Check sheet for the drawn part. Datum: minimum x, y, z corner. Units: mm. A direction names the side the tool comes from. Round coordinates to 2 decimals unless told otherwise and drop trailing zeros. Order: outer loops, then holes, each group sorted by start corner. A loop starts at its lowest first (then second) coordinate and runs counter-clockwise, first axis right, second up. Notation, with made-up numbers: (45.5, 22.5) -> (73.5, 22.5) arc R34 ccw to (73.5, 59.5) -> close; hole circle Ø2 at (53.25, -39.5). An arc over 180 degrees is marked (long way). Answer in a Markdown table with one row per item.
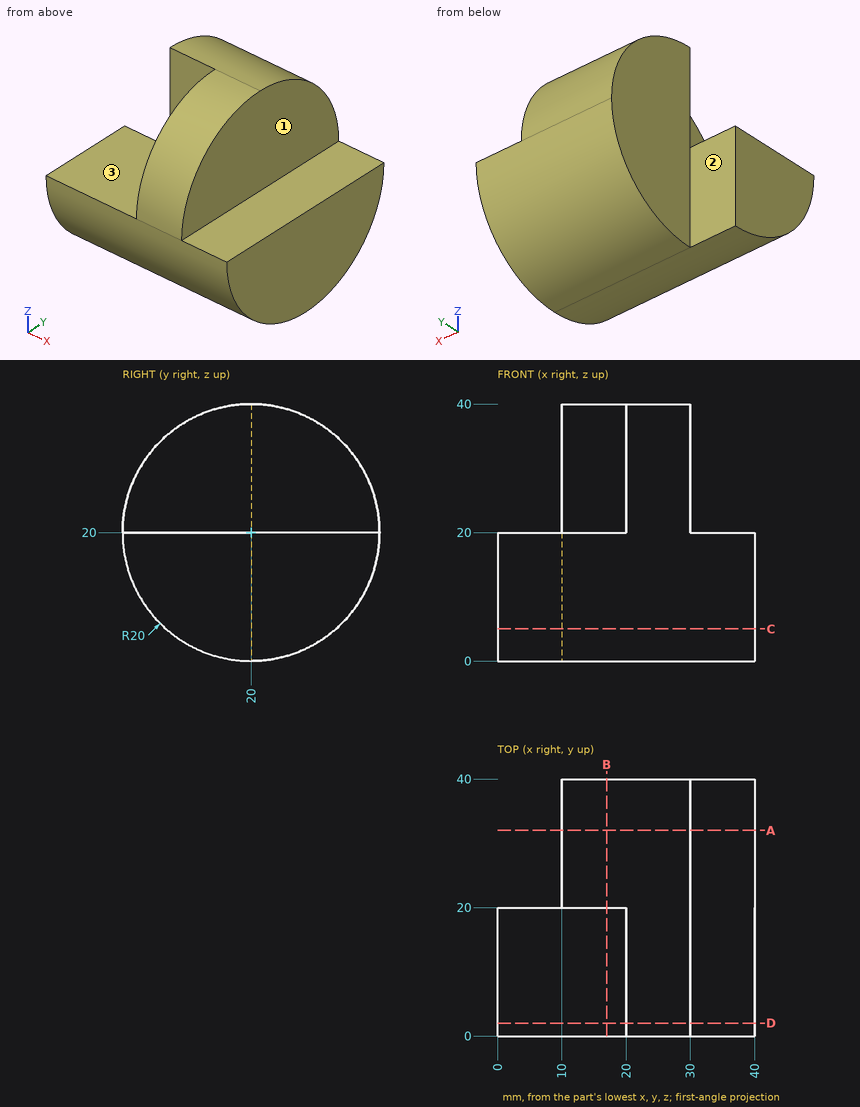
(1) Section check D-D on y = 2. Record the boundary of the cut face in (x, z).
Solutions:
| item | result |
|---|---|
| outline | (0, 11.28) -> (40, 11.28) -> (40, 20) -> (30, 20) -> (30, 28.72) -> (20, 28.72) -> (20, 20) -> (0, 20) -> close |
(2) Section check B-B on x = 17. Record the boundary of the cut face in (y, z), plus the area to 3 significant figures.
Solutions:
| item | result |
|---|---|
| outline | (0, 20) arc R20 ccw (long way) to (20, 40) -> (20, 20) -> close |
| area | 942 mm^2 |
(3) Section check C-C on z = 5. Record the boundary of the cut face in (x, y), plus the area to 3 significant figures.
Solutions:
| item | result |
|---|---|
| outline | (0, 6.77) -> (40, 6.77) -> (40, 33.23) -> (10, 33.23) -> (10, 20) -> (0, 20) -> close |
| area | 926 mm^2 |
(4) Scan lines: probe 1 along X at (y, z) = (35, 12); probe 2 along X at (y, z) = (6.5, 31); probe 3 along Y at (x, z) = (4, 15). Record each from-to range of solid material in increasing order. Write a range as from..to.
Solutions:
| item | result |
|---|---|
| probe 1 | 10..40 |
| probe 2 | 20..30 |
| probe 3 | 0.64..20 |
(5) Tool access check on the marked faces 1, 2 and 3. Record the directions out of +Z, -Z, +X, -X, +Y, -Y that give a thin tool (end or side, any length) a straight path to the whole face; none if there is none.
Solutions:
| item | result |
|---|---|
| face 1 | +Z, +X, +Y, -Y |
| face 2 | +Z, -Z, -X, +Y |
| face 3 | +Z, -X, -Y |
(6) Section check A-A on y = 32. Record the boundary of the cut face in (x, z), plus the area to 3 significant figures.
Solutions:
| item | result |
|---|---|
| outline | (10, 4) -> (40, 4) -> (40, 20) -> (30, 20) -> (30, 36) -> (10, 36) -> close |
| area | 800 mm^2 |
(7) Depth check by flat-ended pin: pin 1 Ø3 at (y, z) = (10.5, 32.5) entering from +X; pin 2 Ø16 at (y, z) = (32, 29.5) entering from -X; pin 3 Ø5 at (x, y) = (35, 20) entering from +Z. Enter the tip coordinate at first touch or a pass-through.
Solutions:
| item | result |
|---|---|
| pin 1 | x = 30 |
| pin 2 | x = 10 |
| pin 3 | z = 20 |
